Here's how the part is built. I have some questions about the finished solid (model axes, mm). A direction names the side the tool comes from. Round coordinates to 2 decimals unless told otherwise and drop trailing zeros. Order: outer loops, then holes, each group sorted by start corner. A loop starts at its lowest first (then second) coordinate and runs counter-clockwise, first axis right, second up. Notation, with made-up numbers: (81, -27.5) -> (100, -27.5) arc R14 cw to (100, -19.5) -> close; hole circle Ø10 at (15, 59.25). An arc over 180 degrees is marked (long way). Use a Markdown table: item, result. Add a question column.
(1) I want a section at B-B, the plane x = -2. Please give me the cut outline in (y, z).
(2) I'm going to push flat-ended pins straight in: P1, Ø0.6, axis at x = -3, y = -0.5, coming from the +Z side; P2, Ø1.8, axis at x = -1.5, z = -2, coming from the -Y side; P3, Ø0.6, axis at x = -3.5, y = -0.5, coming from the -Z side. Where does each tip first touch, or does it pass through?
(3) I want a section at C-C, the plane z = -3. Please give me the cut outline in (x, y).
(4) If I drill on probe 1 along Z at (x, y) = (-5.25, -0.2); probe 2 along Z at (x, y) = (-1.5, 2.05); probe 3 along Z at (x, y) = (-1.75, 1.35), over which ranges is the centre line in solid material (lowest first)?
(5) I want a section at A-A, the plane y = -0.4. Please give me the cut outline in (x, z), then the cut area to 3 significant figures.
(6) On a 3-axis mill with a long thin cutter (end or side, diameter ignored), from which of +Z, -Z, +X, -X, +Y, -Y can I reach the whole of each face in a straight line? I mean faces 1 (the face through (-3, 0, -28)), 2 (the face through (-3, 0, -11)), 3 (the face through (-3, -0.762, -9)), 4 (the face through (-2.3, 0, -4.3)). Say none if no direction works.
(7) I want a section at D-D, the plane x = -0.5. Please give me the cut outline in (y, z).
Autodesk Inventor part; units mm, degrees
ref_plane "YZ Plane" through (0, 0, 0) normal (1, 0, 0) x (0, 1, 0)
ref_plane "XZ Plane" through (0, 0, 0) normal (0, 1, 0) x (-1, 0, 0)
ref_plane "XY Plane" through (0, 0, 0) normal (0, 0, 1) x (1, 0, 0)
sketch "Sketch1" plane through (0, 0, 0) normal (0, 1, 0) x (-1, 0, 0)
  line L0 (0, 0) -> (6.096, 0)
  line L1 (6.096, 0) -> (6.096, -32.6136)
  line L2 (6.096, -32.6136) -> (0, -32.6136)
  line L3 (0, -32.6136) -> (0, 0)
  dimension "d0" = 6.096
  dimension "d1" = 32.6136
extrude "Extrusion1" add sketch "Sketch1" along normal blind 2.54
sketch "Sketch2" plane through (0, 0, 0) normal (0, -1, 0) x (1, 0, 0)
  line L0 (0, 0) -> (0, -32.6136)
  line L1 (0, -7.1628) -> (-6.096, -7.1628)
  line L2 (-6.096, -7.1628) -> (-6.096, -10.2108)
  line L3 (-6.096, -10.2108) -> (0, -10.2108)
  line L4 (0, -10.2108) -> (0, -7.1628)
  line L5 (0, -12.2428) -> (-6.096, -12.2428)
  line L6 (-6.096, -12.2428) -> (-6.096, -15.2908)
  line L7 (-6.096, -15.2908) -> (0, -15.2908)
  line L8 (0, -15.2908) -> (0, -12.2428)
  line L9 (0, -17.3228) -> (-6.096, -17.3228)
  line L10 (-6.096, -17.3228) -> (-6.096, -20.3708)
  line L11 (-6.096, -20.3708) -> (0, -20.3708)
  line L12 (0, -20.3708) -> (0, -17.3228)
  line L13 (0, -22.4028) -> (-6.096, -22.4028)
  line L14 (-6.096, -22.4028) -> (-6.096, -25.4508)
  line L15 (-6.096, -25.4508) -> (0, -25.4508)
  line L16 (0, -25.4508) -> (0, -22.4028)
  line L17 (-3.048, -10.2108) -> (-3.048, -12.2428) construction
  line L18 (-3.048, -15.2908) -> (-3.048, -17.3228) construction
  line L19 (-3.048, -20.3708) -> (-3.048, -22.4028) construction
  line L20 (-6.096, 0) -> (-6.096, -32.6136) construction
  line L21 (-6.096, 0) -> (0, 0) construction
  line L22 (0, -7.1628) -> (0, 0) construction
  line L23 (0, -32.6136) -> (0, -25.4508) construction
  dimension "d4" = 3.048
  dimension "d13" = 2.032
extrude "Extrusion2" add sketch "Sketch2" along normal blind 0.762
sketch "Sketch3" plane through (0, 0, 0) normal (0, -1, 0) x (1, 0, 0)
  line L0 (0, -7.1628) -> (-6.096, -7.1628) construction
  line L1 (-6.096, -7.1628) -> (-6.096, -10.2108) construction
  line L2 (-6.096, -10.2108) -> (0, -10.2108) construction
  line L3 (0, -10.2108) -> (0, -7.1628) construction
  line L4 (0, -22.4028) -> (-6.096, -22.4028) construction
  line L5 (-6.096, -22.4028) -> (-6.096, -25.4508) construction
  line L6 (-6.096, -25.4508) -> (0, -25.4508) construction
  line L7 (0, -25.4508) -> (0, -22.4028) construction
  circle A0 centre (-3.048, -2.5908) radius 1.7145
  circle A1 centre (-3.048, -30.0228) radius 1.7145
  line L8 (0, -7.1628) -> (-6.096, -7.1628)
  line L9 (-6.096, -25.4508) -> (0, -25.4508)
  point P0 (0, 0)
  point P1 (-3.048, -7.1628)
  point P2 (-3.048, -25.4508)
  dimension "d7" = 4.572
  dimension "d8" = 4.572
  dimension "d9" = 3.429
  dimension "d10" = 3.429
extrude "Extrusion3" cut sketch "Sketch3" against normal through all
equation "\"d8\" = d7"
equation "\"d10\" = d9"
properties part number "ContactPress" material "ABS Plastic"
Taken from the geometry:
| question | item | result |
|---|---|---|
| 1 | outline | (-0.76, -25.45) -> (0, -25.45) -> (0, -28.67) -> (2.54, -28.67) -> (2.54, -3.95) -> (0, -3.95) -> (0, -7.16) -> (-0.76, -7.16) -> (-0.76, -10.21) -> (0, -10.21) -> (0, -12.24) -> (-0.76, -12.24) -> (-0.76, -15.29) -> (0, -15.29) -> (0, -17.32) -> (-0.76, -17.32) -> (-0.76, -20.37) -> (0, -20.37) -> (0, -22.4) -> (-0.76, -22.4) -> close; (0, -32.61) -> (2.54, -32.61) -> (2.54, -31.38) -> (0, -31.38) -> close; (0, -1.23) -> (2.54, -1.23) -> (2.54, 0) -> (0, 0) -> close |
| 2 | P1 | stops at z = -7.16 |
| 2 | P2 | stops at y = 0 |
| 2 | P3 | stops at z = -25.45 |
| 3 | outline | (-6.1, 0) -> (-4.71, 0) -> (-4.71, 2.54) -> (-6.1, 2.54) -> close; (-1.38, 0) -> (0, 0) -> (0, 2.54) -> (-1.38, 2.54) -> close |
| 4 | probe 1 | z = -25.45 to -22.4, -20.37 to -17.32, -15.29 to -12.24, -10.21 to -7.16 |
| 4 | probe 2 | z = -32.61 to -30.76, -29.29 to -3.33, -1.85 to 0 |
| 4 | probe 3 | z = -32.61 to -31.14, -28.9 to -3.71, -1.47 to 0 |
| 5 | outline | (-6.1, -25.45) -> (0, -25.45) -> (0, -22.4) -> (-6.1, -22.4) -> close; (-6.1, -20.37) -> (0, -20.37) -> (0, -17.32) -> (-6.1, -17.32) -> close; (-6.1, -15.29) -> (0, -15.29) -> (0, -12.24) -> (-6.1, -12.24) -> close; (-6.1, -10.21) -> (0, -10.21) -> (0, -7.16) -> (-6.1, -7.16) -> close |
| 5 | area | 74.3 mm2 |
| 6 | face 1 | -Z, +X, -X, -Y |
| 6 | face 2 | +X, -X, -Y |
| 6 | face 3 | +Z, -Z, +X, -X, -Y |
| 6 | face 4 | +Z, +X, -X, -Y |
| 7 | outline | (-0.76, -25.45) -> (0, -25.45) -> (0, -32.61) -> (2.54, -32.61) -> (2.54, 0) -> (0, 0) -> (0, -7.16) -> (-0.76, -7.16) -> (-0.76, -10.21) -> (0, -10.21) -> (0, -12.24) -> (-0.76, -12.24) -> (-0.76, -15.29) -> (0, -15.29) -> (0, -17.32) -> (-0.76, -17.32) -> (-0.76, -20.37) -> (0, -20.37) -> (0, -22.4) -> (-0.76, -22.4) -> close |
